The listing builds one solid part. Answer for the finished solid, in the listing's coordinates (mm). A direction names the side the tool comes from. Give positions to 0.01 mm unless a question says otherwise; leave off trailing zeros. Return JSON: item names as keys, results as strings.
from build123d import *

# Parameters (mm, degrees)
EXTRUDE_1_DEPTH         = 290
HOLE_WIZARD_4_5_4_5_1_D = 4.5
HOLE_WIZARD_4_5_4_5_2_D = 4.5
HOLE_WIZARD_4_5_4_5_3_D = 4.5
HOLE_WIZARD_4_5_4_5_4_D = 4.5


with BuildPart() as part:
    # Sketch1 → 凸台-拉伸1 (new body)
    with BuildSketch(Plane.XY):
        with BuildLine():
            Line((-9, 40), (-4.15, 40))
            Line((-4.15, 40), (-4.15, 37))
            Line((-4.15, 37), (-7.05, 37))
            Line((-7.05, 37), (-7.05, 30))
            Line((-7.05, 30), (7.05, 30))
            Line((7.05, 30), (7.05, 37))
            Line((7.05, 37), (4.15, 37))
            Line((4.15, 37), (4.15, 40))
            Line((4.15, 40), (9, 40))
            ThreePointArc((9, 40), (9.707106781, 39.707106781), (10, 39))
            Line((10, 39), (10, 24.15))
            Line((10, 24.15), (6, 24.15))
            Line((6, 24.15), (6, 27.05))
            Line((6, 27.05), (0, 27.05))
            Line((0, 27.05), (0, 24.15))
            Line((0, 24.15), (-4, 24.15))
            Line((-4, 24.15), (-4, 15.85))
            Line((-4, 15.85), (0, 15.85))
            Line((0, 15.85), (0, 12.95))
            Line((0, 12.95), (6, 12.95))
            Line((6, 12.95), (6, 15.85))
            Line((6, 15.85), (10, 15.85))
            Line((10, 15.85), (10, -15.85))
            Line((10, -15.85), (6, -15.85))
            Line((6, -15.85), (6, -12.95))
            Line((6, -12.95), (0, -12.95))
            Line((0, -12.95), (0, -15.85))
            Line((0, -15.85), (-4, -15.85))
            Line((-4, -15.85), (-4, -24.15))
            Line((-4, -24.15), (0, -24.15))
            Line((0, -24.15), (0, -27.05))
            Line((0, -27.05), (6, -27.05))
            Line((6, -27.05), (6, -24.15))
            Line((6, -24.15), (10, -24.15))
            Line((10, -24.15), (10, -39))
            ThreePointArc((10, -39), (9.707106781, -39.707106781), (9, -40))
            Line((9, -40), (4.15, -40))
            Line((4.15, -40), (4.15, -37))
            Line((4.15, -37), (7.05, -37))
            Line((7.05, -37), (7.05, -30))
            Line((7.05, -30), (-7.05, -30))
            Line((-7.05, -30), (-7.05, -37))
            Line((-7.05, -37), (-4.15, -37))
            Line((-4.15, -37), (-4.15, -40))
            Line((-4.15, -40), (-9, -40))
            ThreePointArc((-9, -40), (-9.707106781, -39.707106781), (-10, -39))
            Line((-10, -39), (-10, -4.15))
            Line((-10, -4.15), (-6, -4.15))
            Line((-6, -4.15), (-6, -7.05))
            Line((-6, -7.05), (0, -7.05))
            Line((0, -7.05), (0, -4.15))
            Line((0, -4.15), (4, -4.15))
            Line((4, -4.15), (4, 4.15))
            Line((4, 4.15), (0, 4.15))
            Line((0, 4.15), (0, 7.05))
            Line((0, 7.05), (-6, 7.05))
            Line((-6, 7.05), (-6, 4.15))
            Line((-6, 4.15), (-10, 4.15))
            Line((-10, 4.15), (-10, 39))
            ThreePointArc((-10, 39), (-9.707106781, 39.707106781), (-9, 40))
        make_face()
    extrude(amount=EXTRUDE_1_DEPTH)

    # Ø4.5 (4.5) 直径孔1 (through all)
    with Locations(Plane.ZY.offset(10)):
        with Locations((10, 20)):
            Hole(HOLE_WIZARD_4_5_4_5_1_D / 2)

    # Ø4.5 (4.5) 直径孔2 (through all)
    with Locations(Plane.ZY.offset(10)):
        with Locations((280, 20)):
            Hole(HOLE_WIZARD_4_5_4_5_2_D / 2)

    # Ø4.5 (4.5) 直径孔3 (through all)
    with Locations(Plane.ZY.offset(10)):
        with Locations((10, -20)):
            Hole(HOLE_WIZARD_4_5_4_5_3_D / 2)

    # Ø4.5 (4.5) 直径孔4 (through all)
    with Locations(Plane.ZY.offset(10)):
        with Locations((280, -20)):
            Hole(HOLE_WIZARD_4_5_4_5_4_D / 2)


solid = part.part
(1) Given pin 1 (3 mm diameter, centred on x = 0.5, z = 50, fed in from -Y); pin 2 (6 mm diameter, centred on y = -20, z = 280, fed in from +X), each flat-ended and moving along its own axis, determine where each tip first touches the part or whether it passes through.
Values follow:
{"pin 1": "y = -30", "pin 2": "x = -4"}
(2) Straight lines are drawn through the part: line 1 along Y through (x, z) = (8.25, 18.5); line 2 along Y through (x, z) = (0.25, 115); line 3 along Y through (x, z) = (-3.25, 35). For each, find the intervals that lie inside material, in ascending order.
Values follow:
{"line 1": "-40 to -24.15, -15.85 to 15.85, 24.15 to 40", "line 2": "-30 to -27.05, -12.95 to -4.15, 4.15 to 12.95, 27.05 to 30", "line 3": "-30 to -24.15, -15.85 to -7.05, 7.05 to 15.85, 24.15 to 30"}
(3) A tool of negligible diameter and unlimited length cuts with its end or side. For faces 1 (the flat face through (3, -12.95, 143)), 2 (the flat face through (-10, 21, 143)), 3 (the flat face through (-4, -20, 143)), from which of +Z, -Z, +X, -X, +Y, -Y can it reach the whole face along a straight path? Write none if from no direction.
Values follow:
{"face 1": "+Z, -Z", "face 2": "+Z, -Z, -X, +Y, -Y", "face 3": "+Z, -Z, +X"}
(4) Determine the mould class of faces 4 (the flat face through (-10, -22, 143)), 5 (the flat face through (7.05, -34, 143)), 6 (the flat face through (7, 40, 143)), 7 (the flat face through (10, 0, 143)) for opening direction X: released by +X, released by -X, zero draft, split by the parting line, or undercut.
Values follow:
{"face 4": "released by -X", "face 5": "undercut", "face 6": "zero draft", "face 7": "released by +X"}
